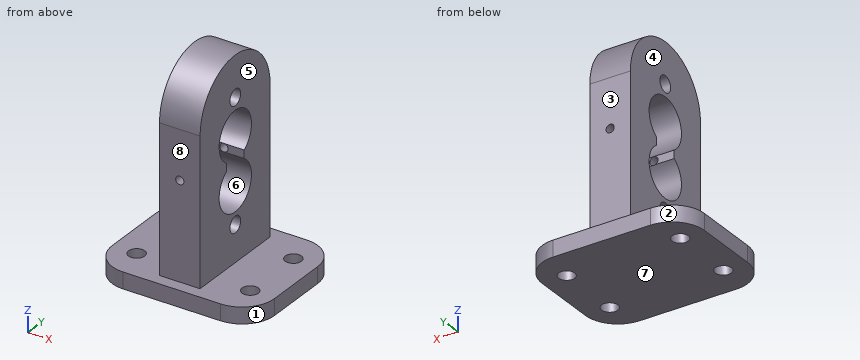
Autodesk Inventor part; units mm, degrees
ref_plane "Arbeitsebene2" through (5, 0, 0) normal (1, 0, 0) x (0, 1, 0)
ref_plane "Arbeitsebene3" through (0, 4, 0) normal (0, 1, 0) x (-1, 0, 0)
ref_plane "XY Plane" through (0, 0, 0) normal (0, 0, 1) x (1, 0, 0)
sketch "Skizze1" plane through (0, 0, 0) normal (0, 0, 1) x (1, 0, 0)
  line L0 (0, 8) -> (10, 8)
  line L1 (10, 8) -> (10, 0)
  line L2 (10, 0) -> (0, 0)
  line L3 (0, 0) -> (0, 8)
  dimension "d0" = 8
  dimension "d1" = 10
extrude "Extrusion1" add sketch "Skizze1" along normal mid plane 1
ref_plane "Arbeitsebene2" through (5, 0, 0) normal (1, 0, 0) x (0, 1, 0)
sketch "Skizze3" plane through (5, 0, 0) normal (1, 0, 0) x (0, 1, 0)
  line L0 (8, 0.5) -> (0, 0.5)
  line L1 (0.7344, 0.5) -> (7.2344, 0.5)
  line L2 (7.2344, 0.5) -> (7.2344, 9.5)
  line L3 (0.7344, 9.5) -> (0.7344, 0.5)
  arc A0 (7.2344, 9.5) -> (0.7344, 9.5) centre (3.9844, 9.5) ccw
  line L4 (0, -0.5) -> (8, -0.5)
  point P0 (0, 0)
  point P1 (3.9844, -0.5)
  dimension "d5" = 6.5
  dimension "d6" = 10
extrude "Extrusion2" add sketch "Skizze3" along normal mid plane 2.5
sketch "Skizze4" plane through (6.25, 0, 0) normal (1, 0, 0) x (0, 0, -1)
  line L0 (-6.75, 3.1708) -> (-6.25, 3.1708)
  line L1 (-6.75, 4.8292) -> (-6.25, 4.8292)
  arc A0 (-6.75, 4.8292) -> (-6.75, 3.1708) centre (-8, 4) ccw
  arc A1 (-6.25, 3.1708) -> (-6.25, 4.8292) centre (-5, 4) ccw
  line L2 (-0.5, 0) -> (-0.5, 8)
  point P0 (0, 0)
  point P1 (-0.5, 4)
  dimension "d9" = 1.5
  dimension "d10" = 0.5
  dimension "d11" = 4.5
  dimension "d12" = 3
extrude "Extrusion3" cut sketch "Skizze4" against normal blind 2.5
sketch "Skizze5" plane through (6.25, 0, 0) normal (1, 0, 0) x (0, 0, -1)
  arc A0 (-6.25, 3.1708) -> (-6.25, 4.8292) centre (-5, 4) ccw
  point P0 (0, 0)
  point P1 (-2.75, 4)
  point P2 (-3.5, 4)
  point P3 (-3.5, 4)
  dimension "d15" = 0.75
hole "Bohrung1" at (6.25, 4, 2.75) direction (-1, 0, 0) diameter 1 end through all
sketch "Skizze6" plane through (6.25, 0, 0) normal (1, 0, 0) x (0, 0, -1)
  arc A0 (-6.75, 4.8292) -> (-6.75, 3.1708) centre (-8, 4) ccw
  point P0 (0, 0)
  point P1 (-10.25, 4)
  point P2 (-9.5, 4)
  point P3 (-9.5, 4)
  dimension "d23" = 0.75
hole "Bohrung2" at (6.25, 4, 10.25) direction (-1, 0, 0) diameter 1 end through all
ref_plane "Arbeitsebene3" through (0, 4, 0) normal (0, 1, 0) x (-1, 0, 0)
sketch "Skizze7" plane through (0, 4, 0) normal (0, 1, 0) x (-1, 0, 0)
  circle A0 centre (-5, 6.4964) radius 0.2536
  line L0 (-6.25, 6.75) -> (-3.75, 6.75)
  point P0 (0, 0)
  point P1 (-5, 6.75)
  dimension "d32" = 0.5072
extrude "Extrusion4" cut sketch "Skizze7" along normal through all both and the other way through all
fillet "Rundung1" radius 2 4 edges at (10, 8, 0) (10, 0, 0) (0, 8, 0) (0, 0, 0)
sketch "Skizze8" plane through (0, 0, 0.5) normal (0, 0, 1) x (1, 0, 0)
  line L0 (10, 2) -> (10, 6)
  line L1 (10, 4) -> (0, 4) construction
  line L2 (2, 0) -> (8, 0)
  line L3 (5, 0) -> (5, 8) construction
  line L4 (2, 8) -> (8, 8)
  point P0 (0, 0)
  point P1 (8.5, 2)
  point P2 (1.5, 2)
  point P3 (1.5, 6)
  point P4 (8.5, 6)
  dimension "d36" = 7
  dimension "d37" = 4
hole "Bohrung3" at (8.5, 2, 0.5) at (1.5, 2, 0.5) at (1.5, 6, 0.5) at (8.5, 6, 0.5) direction (0, 0, -1) diameter 1 end through all
properties part number "grave" material "Stahl, galvanisiert"
Work out the finished part from the listing and answer in its coordinate system (mm). Face numbers are marked on the shaded views. A direction names the side the tool comes from. Give positions to 0.01 mm unless a question says otherwise; leave off trailing zeros. Write each loop counter-clockwise with the first axis right and the second up, starting at its lowest first coordinate (ties: lowest second). Pieces come first, ordered by that corner, then holes.
(1) Which of the six approach directions +Z, -Z, +X, -X, +Y, -Y give full straight-line access (tool end or side, diameter ignored) to the marked faces 1, 2, 3, 4 and 5?
Final values:
face 1: +Z, -Z, +X, -Y
face 2: +Z, -Z, -X, +Y
face 3: +Z, +X, -X, +Y
face 4: +Z, -X, +Y, -Y
face 5: +Z, +X, +Y, -Y
(2) The part is cut by section B-B on y = 1.75. Write down the section's boundary in (x, z), plus the area to 3 significant figures.
Final values:
outline: (0.02, -0.5) - (1.07, -0.5) - (1.07, 0.5) - (0.02, 0.5) - close; (1.93, -0.5) - (8.07, -0.5) - (8.07, 0.5) - (6.25, 0.5) - (6.25, 11.86) - (3.75, 11.86) - (3.75, 0.5) - (1.93, 0.5) - close; (8.93, -0.5) - (9.98, -0.5) - (9.98, 0.5) - (8.93, 0.5) - close; hole circle Ø0.51 at (5, 6.5)
area: 36.4 mm2
(3) Straight lines are drawn through the part: line 1 (Z direction, x = 4.8, y = 4); line 2 (Y direction, x = 1.5, z = 0); line 3 (Y direction, x = 4.55, z = 2.75). For each, find the intervals that lie inside material, in ascending order.
Final values:
line 1: z = -0.5 to 2.25, 3.25 to 3.5, 9.5 to 9.75, 10.75 to 12.75
line 2: y = 0.06 to 1.5, 2.5 to 5.5, 6.5 to 7.94
line 3: y = 0.73 to 3.5, 4.5 to 7.23
(4) The part is cut by section C-C on x = 4.25. Write down the section's boundary in (y, z).
Final values:
outline: (0, -0.5) - (8, -0.5) - (8, 0.5) - (7.23, 0.5) - (7.23, 9.5) arc R3.25 ccw to (0.73, 9.5) - (0.73, 0.5) - (0, 0.5) - close; hole (3.17, 6.25) arc R1.5 ccw (long way) to (4.83, 6.25) - (4.83, 6.75) arc R1.5 ccw (long way) to (3.17, 6.75) - close; hole circle Ø1 at (4, 2.75); hole circle Ø1 at (4, 10.25)
(5) The mould has two halves that part along Z. Classify the marked faces 6, 7 and 8: pulls with the +Z half, pulls with the -Z half, needs draft (parallel to the pull), parting line crosses it, or undercut.
Final values:
face 6: undercut
face 7: pulls with the -Z half
face 8: needs draft
(6) The part is cut by section D-D on y = 3.75. Write down the section's boundary in (x, z), plus the area to 3 significant figures.
Final values:
outline: (0, -0.5) - (10, -0.5) - (10, 0.5) - (6.25, 0.5) - (6.25, 2.32) - (3.75, 2.32) - (3.75, 0.5) - (0, 0.5) - close; (3.75, 3.18) - (6.25, 3.18) - (6.25, 3.52) - (3.75, 3.52) - close; (3.75, 9.48) - (6.25, 9.48) - (6.25, 9.82) - (3.75, 9.82) - close; (3.75, 10.68) - (6.25, 10.68) - (6.25, 12.74) - (3.75, 12.74) - close
area: 21.4 mm2
(7) Flat-ended cylindrical pins translate along their axes: pin 1 Ø2 at (x, z) = (4.5, 6.5) entering from -Y; pin 2 Ø3 at (y, z) = (5.5, 11) entering from -X; pin 3 Ø1 at (y, z) = (1.5, 8) entering from +X. Find the tip coordinate at first contact, or state that the pin passes through.
Final values:
pin 1: stops at y = 0.73
pin 2: stops at x = 3.75
pin 3: stops at x = 6.25
(8) The part is cut by section A-A on z = 2.75. Write down the section's boundary in (x, y).
Final values:
outline: (3.75, 0.73) - (6.25, 0.73) - (6.25, 3.5) - (3.75, 3.5) - close; (3.75, 4.5) - (6.25, 4.5) - (6.25, 7.23) - (3.75, 7.23) - close
